Model file for the job. Use its own axes, mm. Give positions to 0.01 mm unless a question says otherwise; leave off trailing zeros. Write each loop counter-clockwise with the first axis right and the second up, starting at its lowest first coordinate (ties: lowest second). Pieces come first, ordered by that corner, then holes. Notation, with made-up numbers: (25, 15) - (78, 15) arc R29 cw to (78, 35) - close; hole circle Ø1 at (-35.5, 62). An arc over 180 degrees is marked (long way). One line per item, written item: value. Start each with the question number.
(1) Cut at D-D, the plane x = -2. List the corners of the cut face in (y, z), and give its area (4 significant figures).
(2) Drop flat-ended pins along their axis: P1, Ø1.6, axis at x = 17, z = 18.5, coming from the -Y side; P2, Ø1.5, axis at y = -19.5, z = 26, coming from the -X side; P3, Ø0.8, axis at y = -19.5, z = 15, coming from the +X side. Give the stop position or say it passes through.
(3) Cut at A-A, the plane x = 3. List the corners of the cut face in (y, z).
(4) Cut at C-C, the plane z = 14.5. List the corners of the cut face in (x, y).
(5) Probe L1, parallel to Z at x = 0.5, y = -17.8; L2, parallel to X at y = -19.7, z = 14. List the from-to ranges inside material, lowest first.
(6) Cut at B-B, the plane y = -17.95. List the corners of the cut face in (x, z).
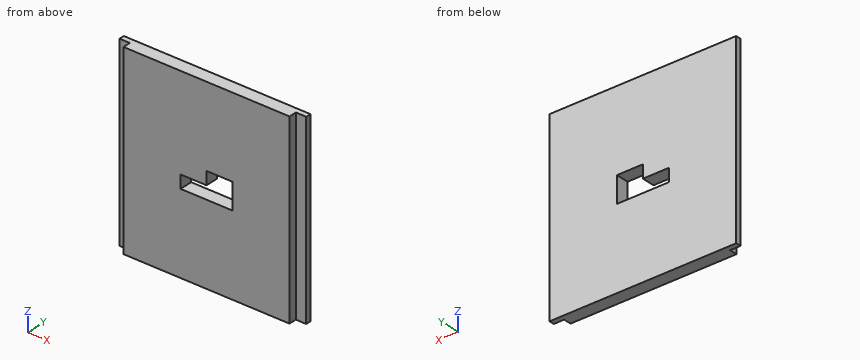
from build123d import *

# Parameters (mm, degrees)
SKETCH021_W                    = 32
SKETCH021_H                    = 36
EXTRUDE019_DEPTH               = 1.5
SKETCH020_W                    = 36
SKETCH020_H                    = 36
EXTRUDE018_DEPTH               = 1
FUSION011_PLACEMENT_ANGLE      = 90
BASEFEATURE002_PLACEMENT_ANGLE = 90
POCKET002_DEPTH                = 5
BODY003_PLACEMENT_ANGLE        = 90


with BuildPart() as extrude019:
    # Sketch021 (on Face6 of Extrude018) → Extrude019 (new body)
    with BuildSketch(Plane.XY.offset(1)):
        Rectangle(SKETCH021_W, SKETCH021_H)
    extrude(amount=EXTRUDE019_DEPTH)


with BuildPart() as body003:
    # Sketch020 → Extrude018 (new body)
    with BuildSketch(Plane.XY):
        Rectangle(SKETCH020_W, SKETCH020_H)
    extrude(amount=EXTRUDE018_DEPTH)

    # Fusion011: union Extrude019
    add(extrude019.part)


with BuildPart() as body003_1:
    # Fusion011 placement: moved
    add(body003.part.moved(Location((0, -17.5, 20))).rotate(Axis((0, -17.5, 20), (1, 0, 0)), FUSION011_PLACEMENT_ANGLE))


with BuildPart() as body003_2:
    # BaseFeature002 placement: moved
    add(body003_1.part.moved(Location((0, -20, -17.5))).rotate(Axis((0, -20, -17.5), (-1, 0, 0)), BASEFEATURE002_PLACEMENT_ANGLE))

    # Sketch026 (on Face8 of BaseFeature002) → Pocket002 (cut)
    with BuildSketch(Plane.XY.offset(2.5)):
        Polygon((0, 0), (0, 2.5), (5, 2.5), (5, -2.5), (-5, -2.5), (-5, 0), align=None)
    extrude(amount=-POCKET002_DEPTH, mode=Mode.SUBTRACT)


with BuildPart() as body003_3:
    # Body003 placement: moved
    add(body003_2.part.moved(Location((0, -17.5, 20))).rotate(Axis((0, -17.5, 20), (1, 0, 0)), BODY003_PLACEMENT_ANGLE))


solid = body003_3.part
Answers follow:
1. outline: (-20, 2) - (-17.5, 2) - (-17.5, 17.5) - (-20, 17.5) - close; (-20, 20) - (-17.5, 20) - (-17.5, 38) - (-20, 38) - close
1. area: 83.75 mm²
2. P1: stops at y = -18.5
2. P2: stops at x = -16
2. P3: stops at x = 16
3. outline: (-20, 2) - (-17.5, 2) - (-17.5, 17.5) - (-20, 17.5) - close; (-20, 22.5) - (-17.5, 22.5) - (-17.5, 38) - (-20, 38) - close
4. outline: (-18, -18.5) - (-16, -18.5) - (-16, -20) - (16, -20) - (16, -18.5) - (18, -18.5) - (18, -17.5) - (-18, -17.5) - close
5. L1: z = 2 to 17.5, 22.5 to 38
5. L2: x = -16 to 16
6. outline: (-18, 2) - (18, 2) - (18, 38) - (-18, 38) - close; hole (-5, 17.5) - (5, 17.5) - (5, 22.5) - (0, 22.5) - (0, 20) - (-5, 20) - close
